Geometry: final body of the model. Coordinates: model frame, mm. A direction names the side the tool comes from. Give positions to 0.01 mm unless a question says otherwise; leave off trailing zeros. Write each loop counter-clockwise with the first axis right and the second up, starting at its lowest first coordinate (ties: lowest second). Pieces come first, ordered by that corner, then holes. Notation, with made-up numbers: (58.25, -17) - (71.25, -17) arc R12 ccw to (71.25, -5) - close; hole circle Ø3 at (86, 28.5). An arc over 180 degrees is marked (long way). Return JSON: item names as keys, results as strings.
from build123d import *

# Parameters (mm, degrees)
F0_W     = 93
F0_H     = 87
F0_R     = 3
F0_R_2   = 2
F0_R_3   = 3.5
F0_W_2   = 78.25
F0_H_2   = 51.25
F1_DEPTH = 2
F2_R     = 4
F3_DEPTH = 9
F4_R     = 1.5
F5_DEPTH = 25
F6_W     = 26
F6_H     = 87
F6_W_2   = 5
F6_H_2   = 25.5
F7_DEPTH = 2


# Not quite as in the source:
# - a feature of the source that left no trace in its solid (it failed there, or was rolled back) is left out


with BuildPart() as f1:
    # F0 (on Front) → F1 (new body)
    with BuildSketch(Plane.XZ):
        Rectangle(F0_W, F0_H)
        with Locations((-38.5, -31.5)):
            Circle(F0_R, mode=Mode.SUBTRACT)
        with Locations((3.5, -35.5)):
            Circle(F0_R_2, mode=Mode.SUBTRACT)
        with Locations((18.5, -35.5)):
            Circle(F0_R_2, mode=Mode.SUBTRACT)
        with Locations((36.5, -35.5)):
            Circle(F0_R_3, mode=Mode.SUBTRACT)
        with Locations((-0.875, 8.375)):
            Rectangle(F0_W_2, F0_H_2, mode=Mode.SUBTRACT)
    extrude(amount=F1_DEPTH)

    # F2 (on face) → F3 (join)
    with BuildSketch(Plane(origin=(0, 0, 0), x_dir=(-1, 0, 0), z_dir=(0, 1, 0))):
        with Locations((-44, 41)):
            Circle(F2_R)
        with Locations((44, 41)):
            Circle(F2_R)
        with Locations((44, -25)):
            Circle(F2_R)
        with Locations((-44, -25)):
            Circle(F2_R)
    extrude(amount=F3_DEPTH)

    # F4 (on face) → F5 (cut)
    with BuildSketch(Plane(origin=(0, 9, 0), x_dir=(-1, 0, 0), z_dir=(0, 1, 0))):
        with Locations((-44, 41)):
            Circle(F4_R)
        with Locations((44, 41)):
            Circle(F4_R)
        with Locations((44, -25)):
            Circle(F4_R)
        with Locations((-44, -25)):
            Circle(F4_R)
    extrude(amount=-F5_DEPTH, mode=Mode.SUBTRACT)

    # F6 (on face) → F7 (join)
    with BuildSketch(Plane(origin=(-46.5, 0, 0), x_dir=(0, -1, 0), z_dir=(-1, 0, 0))):
        with Locations((-11, 0)):
            Rectangle(F6_W, F6_H)
        with Locations((-17.3, 8.75)):
            Rectangle(F6_W_2, F6_H_2, mode=Mode.SUBTRACT)
    extrude(amount=F7_DEPTH)


solid = f1.part
Q1. Set-up query: faces 5 (the cylindrical face through (18.066, -0.986, -37.452)), 6 (the flat face through (44, 9, 39)), 7 (the flat face through (-1, 0, -19)). Return all of +Z, -Z, +X, -X, +Y, -Y with unobstructed straight access to the full face (end or side cutting, diameter ignored); none if empty.
Answer key:
{"face 5": "+Y, -Y", "face 6": "+Z, -Z, +X, +Y", "face 7": "+Y"}
Q2. Mould query, pull axis Z, two halves, no side actions, for faces 1 (the cylindrical face through (45.11, 3.58, -23.99)), 2 (the flat face through (-11.3, -0.5, 43.5)), 3 (the flat face through (-42, 9, 41)), 4 (the cylindrical face through (33.92, -0.986, -33.135)). Classes: pulls with the +Z half, pulls with the -Z half, needs draft (parallel to the pull), parting line crosses it, or undercut.
Answer key:
{"face 1": "undercut", "face 2": "pulls with the +Z half", "face 3": "needs draft", "face 4": "undercut"}
Q3. Section query A-A, the plane z = -11.5. Return the cut outline in (x, y), plus the area to 3 significant figures.
Answer key:
{"outline": "(-48.5, -2) - (-40, -2) - (-40, 0) - (-46.5, 0) - (-46.5, 24) - (-48.5, 24) - close; (38.25, -2) - (46.5, -2) - (46.5, 0) - (38.25, 0) - close", "area": "81.5 mm^2"}
Q4. Section query B-B, the plane y = 18. Return the cut outline in (x, z).
Answer key:
{"outline": "(-48.5, -43.5) - (-46.5, -43.5) - (-46.5, -4) - (-48.5, -4) - close; (-48.5, 21.5) - (-46.5, 21.5) - (-46.5, 43.5) - (-48.5, 43.5) - close"}
Q5. Pin query (flat end, axial travel): P1, Ø0.8, axis at x = -43, z = 44, coming from the -Y side; P2, Ø12, axis at y = 7.5, z = 20.5, coming from the +X side; P3, Ø1.6, axis at y = -1, z = -8.5, coming from the +X side. Return the tip coordinate at first contact, or that it passes through.
Answer key:
{"P1": "stops at y = 0", "P2": "stops at x = -46.5", "P3": "stops at x = 46.5"}
Q6. Material intervals for probe 1 along Z at (x, y) = (44, 3.75); probe 2 along Z at (x, y) = (-38.5, -1.6); probe 3 along Z at (x, y) = (18.5, -1.05), sorted ascending. Write a range as [from, to].
Answer key:
{"probe 1": "z = [-29, -26.5], [-23.5, -21], [37, 39.5], [42.5, 45]", "probe 2": "z = [-43.5, -34.5], [-28.5, -17.25], [34, 43.5]", "probe 3": "z = [-43.5, -37.5], [-33.5, -17.25], [34, 43.5]"}
Q7. Section query C-C, the plane x = -16.5. Return the cut outline in (y, z).
Answer key:
{"outline": "(-2, -43.5) - (0, -43.5) - (0, -17.25) - (-2, -17.25) - close; (-2, 34) - (0, 34) - (0, 43.5) - (-2, 43.5) - close"}
Q8. Section query D-D, the plane z = 41. Return the cut outline in (x, y), plus the area to 4 significant figures.
Answer key:
{"outline": "(-48.5, -2) - (-45.5, -2) - (-45.5, 9) - (-46.5, 9) - (-46.5, 24) - (-48.5, 24) - close; (-42.5, -2) - (42.5, -2) - (42.5, 9) - (40, 9) - (40, 0) - (-40, 0) - (-40, 9) - (-42.5, 9) - close; (45.5, -2) - (46.5, -2) - (46.5, 0) - (48, 0) - (48, 9) - (45.5, 9) - close", "area": "302.5 mm^2"}
